Input: part model. Units: mm. Frame: model coordinates. Face numbers are marked on the shaded views. A direction names the side the tool comes from. Give positions to 0.01 mm unless a question says otherwise; leave off trailing zeros. Order: outer loops, then holes, each group sorted by start corner. A loop starts at its lowest first (then second) coordinate and runs counter-clockwise, first axis right, second up. Notation, with made-up numbers: M 52,-39.75 L 82,-39.75 A23 cw 82,-2.75 Z; hole C -19.75,-22 d11. An arc over 180 degrees is marked long. Use a Markdown table: item, result.
Autodesk Fusion 360 part; units mm, degrees
sketch "Sketch1" plane through (0, 0, 0) normal (0, 1, 0) x (1, 0, 0)
  circle A0 centre (0, 0) radius 14.5
  dimension "d1" = 29
extrude "Extrude1" add sketch "Sketch1" along normal blind 37.8
sketch "Sketch2" plane through (0, 37.8, 0) normal (0, 1, 0) x (-1, 0, 0)
  circle A0 centre (0, 0) radius 14.5
  circle A1 centre (0, 0) radius 18.5
  dimension "d4" = 37
extrude "Extrude2" add sketch "Sketch2" along normal blind 22.5 contours A0 | A1
sketch "Sketch3" plane through (0, 60.3, 0) normal (0, 1, 0) x (-1, 0, 0)
  circle A0 centre (0, 0) radius 18.5
  circle A1 centre (0, 6) radius 6
  dimension "d7" = 12
extrude "Extrude3" add sketch "Sketch3" along normal blind 6.3 contours A1
sketch "Sketch4" plane through (0, 66.6, 0) normal (0, 1, 0) x (-1, 0, 0)
  circle A0 centre (0, 6) radius 6
  circle A1 centre (0, 6) radius 3
  dimension "d10" = 6
extrude "Extrude4" add sketch "Sketch4" along normal blind 30 contours A1
sketch "Sketch5" plane through (0, 0, 0) normal (1, 0, 0) x (0, 1, 0)
sketch "Sketch6" plane through (0, 0, 0) normal (1, 0, 0) x (0, 1, 0)
  circle A0 centre (91, 6) radius 1.5
  dimension "d13" = 3
extrude "Extrude5" cut sketch "Sketch6" along normal mid plane 6
sketch "Sketch7" plane through (0, 0, 0) normal (0, -1, 0) x (1, 0, 0)
  circle A0 centre (0, 0) radius 14.5
  circle A1 centre (0, 0) radius 5
  dimension "d16" = 10
extrude "Extrude6" add sketch "Sketch7" along normal blind 2.5 contours A1
sketch "Sketch8" plane through (0, -2.5, 0) normal (0, -1, 0) x (1, 0, 0)
  circle A0 centre (0, 0) radius 5
  circle A1 centre (0, 0) radius 2
  dimension "d19" = 4
extrude "Extrude7" add sketch "Sketch8" along normal blind 4 contours A1
sketch "Sketch9" plane through (0, -6.5, 0) normal (0, -1, 0) x (1, 0, 0)
  circle A0 centre (0, 0) radius 2
  circle A1 centre (0, 0) radius 1
  dimension "d22" = 2
extrude "Extrude8" add sketch "Sketch9" along normal blind 2 contours A1
sketch "Sketch10" plane through (0, 0, 0) normal (1, 0, 0) x (0, 1, 0)
  circle A0 centre (-5, 0) radius 0.75
  dimension "d25" = 1.5
extrude "Extrude9" cut sketch "Sketch10" along normal mid plane 5
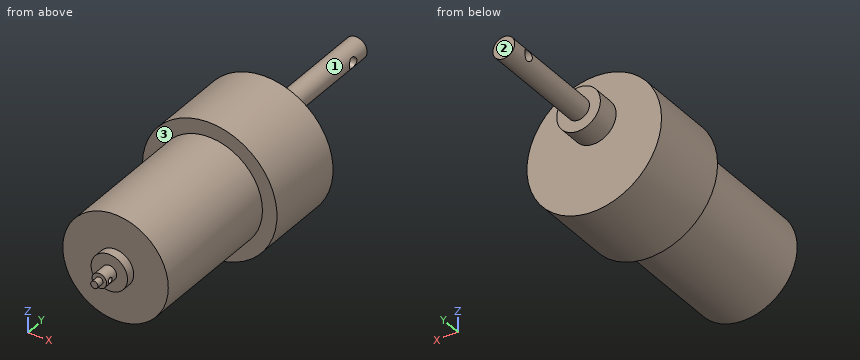
1) Cut plane A-A on x = 0. State how many separate pieces and enclosed holes the cut face has, and give its area (3 significant figures).
Response values:
| item | result |
|---|---|
| separate pieces | 1 |
| enclosed holes | 2 |
| area | 2,220 mm² |
2) First-contact query: pin 1 Ø1 at (x, z) = (-6, -7) entering from -Y; pin 2 Ø4 at (y, z) = (91, 6) entering from -X; pin 3 Ø6 at (x, y) = (-1.5, 20.5) entering from +Z. Flat tips, straight axial feed; report the tip coordinate or a pass-through.
Response values:
| item | result |
|---|---|
| pin 1 | stops at y = 0 |
| pin 2 | stops at x = -3 |
| pin 3 | stops at z = 14.5 |
3) Material intervals for line 1 (Z direction, x = 0, y = 91); line 2 (Y direction, x = 1, z = 6); line 3 (Y direction, x = 0.75, z = 0), sorted ascending. Write a range as from..to.
Response values:
| item | result |
|---|---|
| line 1 | z = 3..4.5, 7.5..9 |
| line 2 | y = 0..89.5, 92.5..96.6 |
| line 3 | y = -8.5..-5.75, -4.25..60.3 |
4) Cut plane D-D on z = -3. Return loops of the section in (x, y).
Response values:
| item | result |
|---|---|
| outline | M -18.26,37.8 L -14.19,37.8 L -14.19,0 L -4,0 L -4,-2.5 L 4,-2.5 L 4,0 L 14.19,0 L 14.19,37.8 L 18.26,37.8 L 18.26,60.3 L -18.26,60.3 Z |
5) Cut plane B-B on z = 6. Return loops of the section in (x, y).
Response values:
| item | result |
|---|---|
| outline | M -17.5,37.8 L -13.2,37.8 L -13.2,0 L 13.2,0 L 13.2,37.8 L 17.5,37.8 L 17.5,60.3 L 6,60.3 L 6,66.6 L 3,66.6 L 3,89.5 L -3,89.5 L -3,66.6 L -6,66.6 L -6,60.3 L -17.5,60.3 Z; M -3,92.5 L 3,92.5 L 3,96.6 L -3,96.6 Z |
6) Cut plane C-C on y = 68.5. Return loops of the section in (x, z), and give its area (3 significant figures).
Response values:
| item | result |
|---|---|
| outline | C 0,6 d6 |
| area | 28.3 mm² |
7) Reachability of the marked faces 1, 2 and 3 from +Z, -Z, +X, -X, +Y, -Y: full face, straight path, thin tool, end or side. Return the list, or none.
Response values:
| item | result |
|---|---|
| face 1 | +Y |
| face 2 | +Z, -Z, +X, -X, +Y |
| face 3 | -Y |
